For this review, take the finished solid that the model builds, in its own axes (mm). Face numbers are marked on the shaded views. A direction names the side the tool comes from. Give positions to 0.01 mm unless a question says otherwise; leave off trailing zeros. Write each loop counter-clockwise with the first axis right and the second up, starting at its lowest first coordinate (ties: lowest second). Pieces come first, ordered by that corner, then holes.
1) Machinability: for the marked faces 1 and 2, which of the approach directions +Z, -Z, +X, -X, +Y, -Y give a long, thin tool a straight path to every point of the face, cutting with its end or side? Answer none if there is none.
2) We need section C-C on y = -2.25. Give the boundary of the cut face in (x, z).
3) We need section B-B on x = 1.27. Give the boundary of the cut face in (y, z), and give its area (3 significant figures).
4) Wall thickness on line 1 along X through (y, z) = (-0.65, 0); line 2 along Y through (x, z) = (0.85, -2.1); line 3 along Z through (x, y) = (1.25, -2.1): over which ranges is each line inside the solid? List them lowest first.
5) We need section D-D on x = 0.2. Give the boundary of the cut face in (y, z).
6) We need section A-A on z = 0. Give the boundary of the cut face in (x, y), and give its area (3 significant figures).
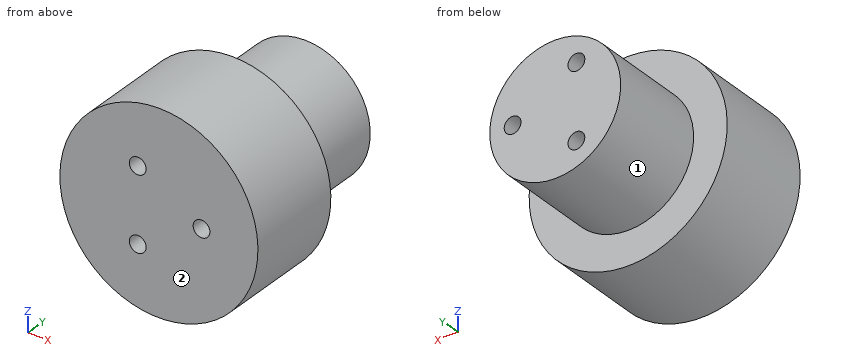
from build123d import *

# Parameters (mm, degrees)
SKETCH_1_R          = 2.95
EXTRUDE_1_DEPTH     = 3
SKETCH_2_R          = 1.95
EXTRUDE_2_DEPTH     = 3
SKETCH_3_R          = 0.25
CUT_EXTRUDE_1_DEPTH = 6


with BuildPart() as part:
    # Эскиз1 → Бобышка-Вытянуть1 (new body)
    with BuildSketch(Plane(origin=(0, 0, 0), x_dir=(1, 0, 0), z_dir=(0, 1, 0))):
        with Locations(Location((0, 0, 0), (0, 0, 270))):
            Circle(SKETCH_1_R)
    extrude(amount=-EXTRUDE_1_DEPTH)

    # Эскиз2 → Бобышка-Вытянуть2 (add)
    with BuildSketch(Plane(origin=(0, 0, 0), x_dir=(1, 0, 0), z_dir=(0, 1, 0))):
        with Locations(Location((0, 0, 0), (0, 0, 270))):
            Circle(SKETCH_2_R)
    extrude(amount=EXTRUDE_2_DEPTH)

    # Эскиз3 → Вырез-Вытянуть1 (cut)
    with BuildSketch(Plane.XZ.offset(3)):
        with Locations(Location((1.27, 0, 0), (0, 0, 270))):
            Circle(SKETCH_3_R)
        with Locations(Location((-0.630957819, 1.102176134, 0), (0, 0, 270))):
            Circle(SKETCH_3_R)
        with Locations(Location((-0.630957819, -1.102176134, 0), (0, 0, 270))):
            Circle(SKETCH_3_R)
    extrude(amount=-CUT_EXTRUDE_1_DEPTH, mode=Mode.SUBTRACT)


solid = part.part
Results list:
1. face 1: +Y
1. face 2: +Z, -Z, +X, -X, -Y
2. outline: circle Ø5.9 at (0, 0); hole circle Ø0.5 at (-0.63, -1.1); hole circle Ø0.5 at (-0.63, 1.1); hole circle Ø0.5 at (1.27, 0)
3. outline: (-3, -2.66) - (0, -2.66) - (0, -1.48) - (3, -1.48) - (3, -0.25) - (-3, -0.25) - close; (-3, 0.25) - (3, 0.25) - (3, 1.48) - (0, 1.48) - (0, 2.66) - (-3, 2.66) - close
3. area: 21.9 mm2
4. line 1: x = -2.95 to 1.02, 1.52 to 2.95
4. line 2: y = -3 to 0
4. line 3: z = -2.67 to -0.25, 0.25 to 2.67
5. outline: (-3, -2.94) - (0, -2.94) - (0, -1.94) - (3, -1.94) - (3, 1.94) - (0, 1.94) - (0, 2.94) - (-3, 2.94) - close
6. outline: (-2.95, -3) - (1.02, -3) - (1.02, 3) - (-1.95, 3) - (-1.95, 0) - (-2.95, 0) - close; (1.52, -3) - (2.95, -3) - (2.95, 0) - (1.95, 0) - (1.95, 3) - (1.52, 3) - close
6. area: 26.4 mm2
